Here's how the part is built. I have some questions about the finished solid (model axes, mm). Face numbers are marked on the shaded views. Give positions to 0.01 mm unless a question says otherwise; leave off trailing zeros. Loops run counter-clockwise (first coordinate to the right, second up) from the corner with the lowest first, then second, coordinate; pieces in that order, holes last. Notation, with made-up numbers: (-4.75, 3) - (20.25, 3) arc R21 ccw to (20.25, 35) - close; hole circle Ø9 at (0, 68.5). An arc over 180 degrees is marked (long way). Use a Markdown table: item, result.
from build123d import *

# Parameters (mm, degrees)
CHAMFER_1_SIZE = 0.2


with BuildPart() as part:
    # Эскиз3 → Повернуть1 (revolve)
    with BuildSketch(Plane.XY):
        with BuildLine():
            Line((0, 2), (4, 2))
            Line((4, 2), (4, 6.5))
            Line((4, 6.5), (2.9, 6.5))
            ThreePointArc((2.9, 6.5), (2, 5.6), (1.1, 6.5))
            Line((1.1, 6.5), (0, 6.5))
            Line((0, 6.5), (0, 2))
        make_face()
    revolve(axis=Axis((7.18815516, 0, 0), (-1, 0, 0)))

    # Фаска1
    chamfer_1_edges = [part.edges().sort_by_distance(p)[0] for p in [
        (4, -2, 0),
        (0, -2, 0),
    ]]
    chamfer(chamfer_1_edges, length=CHAMFER_1_SIZE)


solid = part.part
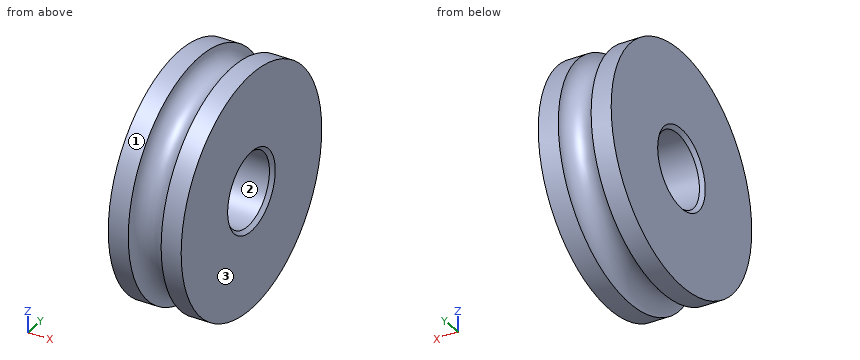
(1) We'd pull the mould along Y, two halves only. Please class the marked faces 1, 2 and 3: pulls with the +Y half, pulls with the -Y half, needs draft (parallel to the pull), parting line crosses it, or undercut.
A:
| item | result |
|---|---|
| face 1 | parting line crosses it |
| face 2 | undercut |
| face 3 | needs draft |
(2) Will these pins go through, and if not, where does the flat tip stop? pin 1 (2 mm diameter, centred on x = 1, y = 3.5, fed in from -Z); pin 2 (1 mm diameter, centred on x = 2, y = -5, fed in from -Z); pin 3 (3 mm diameter, centred on y = 0, z = 0, fed in from +X).
A:
| item | result |
|---|---|
| pin 1 | z = -6 |
| pin 2 | z = -3.33 |
| pin 3 | through |
(3) Suppose I cut it at A-A on y = 0. Write out the boundary of the cut face in (x, z).
A:
| item | result |
|---|---|
| outline | (0, -6.5) - (1.1, -6.5) arc R0.9 cw to (2.9, -6.5) - (4, -6.5) - (4, -2.2) - (3.8, -2) - (0.2, -2) - (0, -2.2) - close; (0, 2.2) - (0.2, 2) - (3.8, 2) - (4, 2.2) - (4, 6.5) - (2.9, 6.5) arc R0.9 cw to (1.1, 6.5) - (0, 6.5) - close |
(4) Suppose I cut it at C-C on x = 0.5. Write out the boundary of the cut face in (y, z), plus the area to 3 significant figures.
A:
| item | result |
|---|---|
| outline | circle Ø13 at (0, 0); hole circle Ø4 at (0, 0) |
| area | 120 mm2 |
(5) Suppose I cut it at D-D on x = 2.55. Write out the boundary of the cut face in (y, z).
A:
| item | result |
|---|---|
| outline | circle Ø11.58 at (0, 0); hole circle Ø4 at (0, 0) |
(6) If I drill on line 1 (Y direction, x = 0.9, z = 0); line 2 (Y direction, x = 2.4, z = 0); line 3 (Z direction, x = 1.4, y = 0), over which ranges is the centre line in solid material (lowest first)?
A:
| item | result |
|---|---|
| line 1 | -6.5 to -2, 2 to 6.5 |
| line 2 | -5.69 to -2, 2 to 5.69 |
| line 3 | -5.83 to -2, 2 to 5.83 |
